Source: CAD feature listing. Evaluate the final solid. Frame: model axes, mm. A direction names the side the tool comes from. Coordinates: 2 decimals unless noted, no trailing zeros. Write each loop counter-clockwise with the first axis right and the second up, starting at its lowest first coordinate (ties: lowest second). Pieces come first, ordered by that corner, then holes. Notation, with made-up numbers: M 80,29 L 85,29 A8 ccw 85,42 Z; hole C 11,-8.75 d3. An arc over 180 degrees is marked long. One line per item, written item: value. Start each with the question number.
Item 1: Pin query (flat end, axial travel): P1, Ø1.6, axis at x = 5, y = -1, coming from the +Z side; P2, Ø2, axis at y = -5.5, z = 5, coming from the +X side; P3, Ø2, axis at x = -5, y = -3, coming from the +Z side. Return the tip coordinate at first contact, or that it passes through.
Item 2: Ray query, L1, parallel to X at y = -6.25, z = 4; L2, parallel to X at y = 0, z = -1.25; L3, parallel to Z at x = -5.75, y = 3.25. Return the intervals inside material, ascending. Write a range as from..to.
Item 3: Cut plane A-A, the plane x = 0. Output: boundary loops of the cut face in (y, z).
Item 4: Mould query, pull axis X, two halves, no side actions, for faces 4 (the flat face through (1, 12, -5)), 5 (the cylindrical face through (-3.7, 0.17, -1.52)), 6 (the cylindrical face through (7.154, 9.859, 2.253)). Classes: released by +X, released by -X, zero draft, split by the parting line, or undercut.
Item 5: Set-up query: faces 1 (the flat face through (1.4, -12, -4.2)), 2 (the flat face through (7, 7.65, -2)), 3 (the cylindrical face through (-6, 0, 0)). Return all of +Z, -Z, +X, -X, +Y, -Y with unobstructed straight access to the full face (end or side cutting, diameter ignored); none if empty.
```python
from build123d import *

# Parameters (mm, degrees)
F0_R       = 7.5
F0_R_2     = 4
F1_DEPTH   = 12
F3_DEPTH   = 24.001
F4_W       = 1.1
F4_H       = 0.7
F6_SIZE2   = 0.5773502692
F6_SIZE    = 1
F6_2_SIZE2 = 0.5773502692
F6_2_SIZE  = 1


with BuildPart() as f1:
    # F0 (on Front) → F1 (new body, symmetric)
    with BuildSketch(Plane.XZ):
        Circle(F0_R)
        Circle(F0_R_2, mode=Mode.SUBTRACT)
    extrude(amount=F1_DEPTH, both=True)

    # F2 (on face) → F3 (cut, through all)
    with BuildSketch(Plane.XZ.offset(12)):
        with BuildLine():
            Line((0.5, 3.9686269666), (0.5, 5.9791303716))
            ThreePointArc((0.5, 5.9791303716), (0, 6), (-0.5, 5.9791303716))
            Line((-0.5, 5.9791303716), (-0.5, 3.9686269666))
            ThreePointArc((-0.5, 3.9686269666), (0, 4), (0.5, 3.9686269666))
        make_face()
        with BuildLine():
            Line((3.1597964307, 2.4526896495), (4.5814370219, 3.8743302407))
            ThreePointArc((4.5814370219, 3.8743302407), (4.2426406871, 4.2426406871), (3.8743302407, 4.5814370219))
            Line((3.8743302407, 4.5814370219), (2.4526896495, 3.1597964307))
            ThreePointArc((2.4526896495, 3.1597964307), (2.8284271247, 2.8284271247), (3.1597964307, 2.4526896495))
        make_face()
        with BuildLine():
            ThreePointArc((5.9791303716, -0.5), (5.9947803225, -0.2502176759), (6, 0))
            ThreePointArc((6, 0), (5.9947803225, 0.2502176759), (5.9791303716, 0.5))
            Line((5.9791303716, 0.5), (3.9686269666, 0.5))
            ThreePointArc((3.9686269666, 0.5), (3.9921490369, 0.2504916502), (4, 0))
            ThreePointArc((4, 0), (3.9921490369, -0.2504916502), (3.9686269666, -0.5))
            Line((3.9686269666, -0.5), (5.9791303716, -0.5))
        make_face()
        with BuildLine():
            ThreePointArc((3.8743302407, -4.5814370219), (4.2426406871, -4.2426406871), (4.5814370219, -3.8743302407))
            Line((4.5814370219, -3.8743302407), (3.1597964307, -2.4526896495))
            ThreePointArc((3.1597964307, -2.4526896495), (2.8284271247, -2.8284271247), (2.4526896495, -3.1597964307))
            Line((2.4526896495, -3.1597964307), (3.8743302407, -4.5814370219))
        make_face()
        with BuildLine():
            ThreePointArc((-0.5, -5.9791303716), (0, -6), (0.5, -5.9791303716))
            Line((0.5, -5.9791303716), (0.5, -3.9686269666))
            ThreePointArc((0.5, -3.9686269666), (0, -4), (-0.5, -3.9686269666))
            Line((-0.5, -3.9686269666), (-0.5, -5.9791303716))
        make_face()
        with BuildLine():
            ThreePointArc((-4.5814370219, -3.8743302407), (-4.2426406871, -4.2426406871), (-3.8743302407, -4.5814370219))
            Line((-3.8743302407, -4.5814370219), (-2.4526896495, -3.1597964307))
            ThreePointArc((-2.4526896495, -3.1597964307), (-2.8284271247, -2.8284271247), (-3.1597964307, -2.4526896495))
            Line((-3.1597964307, -2.4526896495), (-4.5814370219, -3.8743302407))
        make_face()
        with BuildLine():
            Line((-3.9686269666, 0.5), (-5.9791303716, 0.5))
            ThreePointArc((-5.9791303716, 0.5), (-6, 0), (-5.9791303716, -0.5))
            Line((-5.9791303716, -0.5), (-3.9686269666, -0.5))
            ThreePointArc((-3.9686269666, -0.5), (-4, 0), (-3.9686269666, 0.5))
        make_face()
        with BuildLine():
            Line((-2.4526896495, 3.1597964307), (-3.8743302407, 4.5814370219))
            ThreePointArc((-3.8743302407, 4.5814370219), (-4.2426406871, 4.2426406871), (-4.5814370219, 3.8743302407))
            Line((-4.5814370219, 3.8743302407), (-3.1597964307, 2.4526896495))
            ThreePointArc((-3.1597964307, 2.4526896495), (-2.8284271247, 2.8284271247), (-2.4526896495, 3.1597964307))
        make_face()
    extrude(amount=-F3_DEPTH, mode=Mode.SUBTRACT)

    # F4 (on Right) → F5 (revolve, cut)
    with BuildSketch(Plane.YZ):
        with Locations((-8.2, 7.15)):
            Rectangle(F4_W, F4_H)
        with Locations((8.2, 7.15)):
            Rectangle(F4_W, F4_H)
    revolve(axis=Axis((0, -12, 0), (0, -1, 0)), mode=Mode.SUBTRACT)

    # F6
    f6_edges = [f1.edges().sort_by_distance(p)[0] for p in [
        (-7.5, -12, 0),
    ]]
    f6_side = f1.faces().sort_by_distance((-7.287868, -12, 0))[0]
    chamfer(f6_edges, length=F6_SIZE, length2=F6_SIZE2, reference=f6_side)

    # F6#2
    f6_2_edges = [f1.edges().sort_by_distance(p)[0] for p in [
        (-7.5, 12, 0),
    ]]
    f6_2_side = f1.faces().sort_by_distance((-7.5, 10.375, 0))[0]
    chamfer(f6_2_edges, length=F6_2_SIZE, length2=F6_2_SIZE2, reference=f6_2_side)


solid = f1.part
```
From the geometry:
1. P1: stops at z = 6.21
1. P2: stops at x = 6.34
1. P3: stops at z = 6.34
2. L1: x = -6.34..-4.47, -3.29..-0.5, 0.5..3.29, 4.47..6.34
2. L2: x = -7.4..-3.8, 3.8..7.4
2. L3: z = -4.82..-0.5, 0.5..4.82
3. outline: M -12,-6.5 L -11.42,-7.5 L -8.75,-7.5 L -8.75,-6.8 L -7.65,-6.8 L -7.65,-7.5 L 7.65,-7.5 L 7.65,-6.8 L 8.75,-6.8 L 8.75,-7.5 L 11,-7.5 L 12,-6.92 L 12,-6 L -12,-6 Z; M -12,6 L 12,6 L 12,6.92 L 11,7.5 L 8.75,7.5 L 8.75,6.8 L 7.65,6.8 L 7.65,7.5 L -7.65,7.5 L -7.65,6.8 L -8.75,6.8 L -8.75,7.5 L -11.42,7.5 L -12,6.5 Z
4. face 4: zero draft
4. face 5: undercut
4. face 6: split by the parting line
5. face 1: +Z, -Z, +X, -X, -Y
5. face 2: none
5. face 3: +Y, -Y
